Model file for the job. Use its own axes, mm. A direction names the side the tool comes from. Round coordinates to 2 decimals unless told otherwise and drop trailing zeros. Loops run counter-clockwise (first coordinate to the right, second up) from the corner with the lowest first, then second, coordinate; pieces in that order, holes last. Notation, with made-up numbers: M 79.5,85.25 L 115.5,85.25 A15 cw 115.5,113.25 Z; hole C 47.5,51.25 d9. An arc over 180 degrees is marked long. Answer in a Markdown table with one row per item.
from build123d import *

# Parameters (mm, degrees)
F0_W     = 127
F0_H     = 76.2
F1_DEPTH = 25.4
F2_SIZE  = 63.5
F3_W     = 63.5
F3_H     = 25.4
F4_DEPTH = 25.4
F5_SIZE  = 63.5
F6_R     = 12.7
F7_R     = 7.62
F9_D     = 25.4
F11_D    = 25.4


with BuildPart() as f1:
    # F0 (on Top) → F1 (new body)
    with BuildSketch(Plane.XY):
        Rectangle(F0_W, F0_H)
    extrude(amount=F1_DEPTH)

    # F2
    f2_edges = [f1.edges().sort_by_distance(p)[0] for p in [
        (-63.5, -38.1, 12.7),
    ]]
    chamfer(f2_edges, length=F2_SIZE)

    # F3 (on face) → F4 (join)
    with BuildSketch(Plane.XZ.offset(38.1)):
        with Locations((31.75, 12.7)):
            Rectangle(F3_W, F3_H)
    extrude(amount=F4_DEPTH)

    # F5
    f5_edges = [f1.edges().sort_by_distance(p)[0] for p in [
        (63.5, 38.1, 12.7),
    ]]
    chamfer(f5_edges, length=F5_SIZE)

    # F6
    f6_edges = [f1.edges().sort_by_distance(p)[0] for p in [
        (63.5, -63.5, 12.7),
        (0, -63.5, 12.7),
    ]]
    fillet(f6_edges, radius=F6_R)

    # F7
    f7_edges = [f1.edges().sort_by_distance(p)[0] for p in [
        (-63.5, 25.4, 12.7),
        (-63.5, 38.1, 12.7),
        (0, 38.1, 12.7),
        (63.5, -25.4, 12.7),
    ]]
    fillet(f7_edges, radius=F7_R)

    # F9 (through all)
    with Locations(Plane.XY.offset(25.4)):
        with Locations((30.48, -38.1)):
            Hole(F9_D / 2)

    # F11 (through all)
    with Locations(Plane.XY.offset(25.4)):
        with Locations((-25.4, 19.05)):
            Hole(F11_D / 2)


solid = f1.part
1. Saw through at C-C (z = 20). Write the cut outline in (x, y).
Verdict:
| item | result |
|---|---|
| outline | M -63.5,28.56 A7.62 ccw -61.27,23.17 L 0,-38.1 L 0,-50.8 A12.7 ccw 12.7,-63.5 L 50.8,-63.5 A12.7 ccw 63.5,-50.8 L 63.5,-28.56 A7.62 ccw 61.27,-23.17 L 2.23,35.87 A7.62 ccw -3.16,38.1 L -55.88,38.1 A7.62 ccw -63.5,30.48 Z; hole C -25.4,19.05 d25.4; hole C 30.48,-38.1 d25.4 |
2. Wall check: probe 1 along Y at (x, z) = (-25.4, 17.5); probe 2 along Y at (x, z) = (30.48, 12.5); probe 3 along X at (y, z) = (-31, 20.25). Give the ranges that are in metal, low to high.
Verdict:
| item | result |
|---|---|
| probe 1 | y = -12.7 to 6.35, 31.75 to 38.1 |
| probe 2 | y = -63.5 to -50.8, -25.4 to 7.62 |
| probe 3 | x = -7.1 to 19.95, 41.01 to 63.5 |
3. Saw through at B-B (x = -25.4). Write the cut outline in (y, z).
Verdict:
| item | result |
|---|---|
| outline | M -12.7,0 L 6.35,0 L 6.35,25.4 L -12.7,25.4 Z; M 31.75,0 L 38.1,0 L 38.1,25.4 L 31.75,25.4 Z |
4. Tool access for faces 1 (the flat face through (0, -44, 13)), 2 (the cylindrical face through (-0.202, 37.504, 12.878)): list every direction of +Z, -Z, +X, -X, +Y, -Y with a clear straight run to the whole face (end or side of a thin tool).
Verdict:
| item | result |
|---|---|
| face 1 | +Z, -Z, -X, -Y |
| face 2 | +Z, -Z, +X, +Y |
5. Pin check, flat tips, straight feed: pin 1 (8 mm diameter, centred on x = 25, z = 22.5, fed in from +Y); pin 2 (20.5 mm diameter, centred on x = -25.4, y = 19.05, fed in from +Z); pin 3 (1 mm diameter, centred on y = 6.5, z = 8, fed in from +X); pin 4 (1.5 mm diameter, centred on x = 37.5, z = 3, fed in from +Y). Stop position of each tip, or through.
Verdict:
| item | result |
|---|---|
| pin 1 | stops at y = 17.1 |
| pin 2 | passes through |
| pin 3 | stops at x = 32.1 |
| pin 4 | stops at y = 1.35 |
6. Mould opens along X. For faces 3 (the cylindrical face through (-15.322, 11.322, 12.522)), 4 (the flat face through (31, -63.5, 13)), 5 (the cylindrical face through (62.936, -25.679, 12.878)), 6 (the flat face through (-30.2, -7.9, 12.5)) say: +X half, -X half, draft (parallel to the pull), parting line (faces both ways), or undercut.
Verdict:
| item | result |
|---|---|
| face 3 | undercut |
| face 4 | draft |
| face 5 | +X half |
| face 6 | -X half |
7. Saw through at D-D (y = -11). Write the cut outline in (x, z), and give its area (3 significant figures).
Verdict:
| item | result |
|---|---|
| outline | M -27.1,0 L 49.1,0 L 49.1,25.4 L -27.1,25.4 Z |
| area | 1,940 mm² |
8. Saw through at A-A (y = 19.05). Write the cut outline in (x, z), and give its area (3 significant figures).
Verdict:
| item | result |
|---|---|
| outline | M -57.15,0 L -38.1,0 L -38.1,25.4 L -57.15,25.4 Z; M -12.7,0 L 19.05,0 L 19.05,25.4 L -12.7,25.4 Z |
| area | 1,290 mm² |
